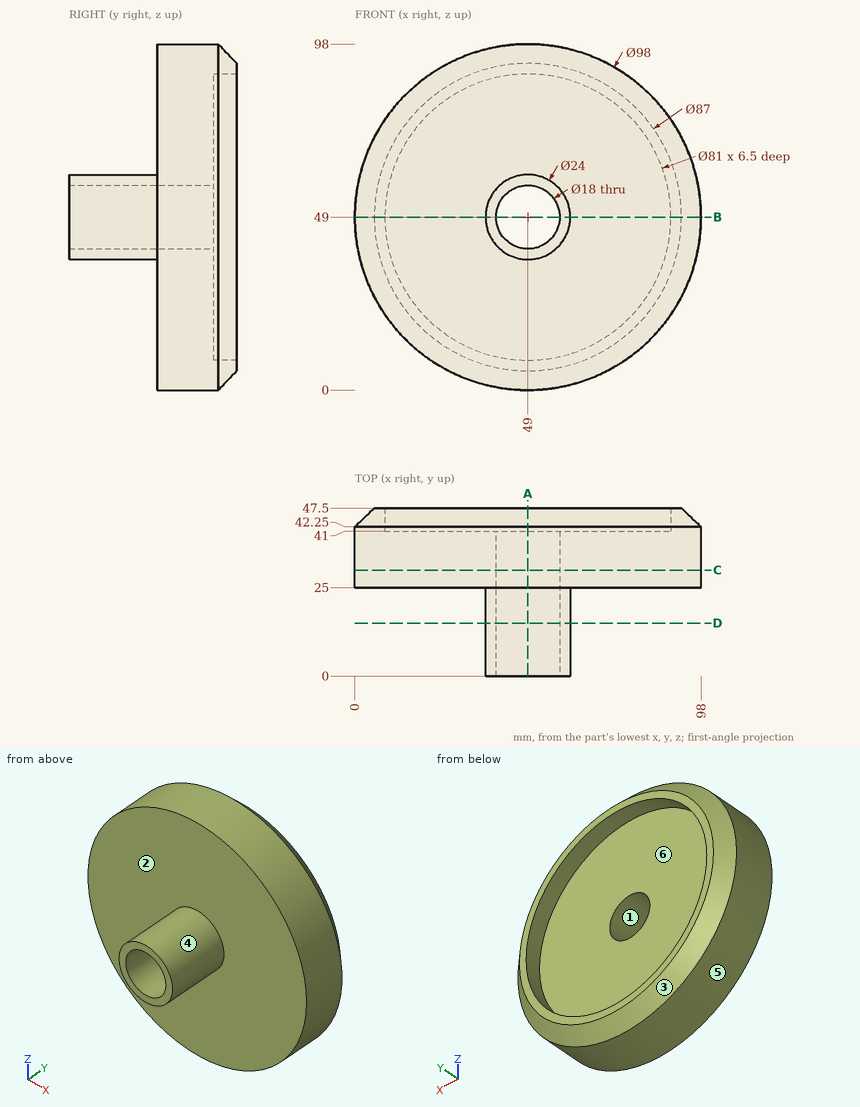
Source: three-view drawing plus pictorial views. Frame: mm from the lowest corner of the part. A direction names the side the tool comes from. Give positions to 0.01 mm unless a question says otherwise; leave off trailing zeros. Order: outer loops, then holes, each group sorted by start corner. A loop starts at its lowest first (then second) coordinate and runs counter-clockwise, first axis right, second up. Notation, with made-up numbers: (6.25, 36.25) -> (20.25, 36.25) arc R8 cw to (20.25, 44.25) -> close; hole circle Ø1 at (41, 70.25). An arc over 180 degrees is marked (long way). Write each question's results on one line, items separated by ' | '. Start each with the question number.
Item 1: Line query: line 1 (X direction, y = 42, z = 49); line 2 (X direction, y = 27, z = 49); line 3 (Y direction, x = 50, z = 64). Output: solid intervals per line, ascending.
Item 2: Cut plane C-C on y = 30. Return the cut outline in (x, z), then the cut area to 3 significant figures.
Item 3: Cut plane A-A on x = 49. Return the cut outline in (y, z).
Item 4: Contact query for flat-ended pins moving along their axis: P1, Ø1.5, axis at y = 27.5, z = 29, coming from the -X side; P2, Ø16, axis at x = 49, z = 49, coming from the +Y side; P3, Ø3, axis at x = 25.5, z = 37.5, coming from the -Y side; P4, Ø24.5, axis at x = 53.5, z = 40, coming from the +Y side. Output: stop coordinate, or through.
Item 5: Cut plane B-B on z = 49. Return the cut outline in (x, y), then the cut area to 3 significant figures.
Item 6: Set-up query: the marked faces 4, 5 and 6. Return all of +Z, -Z, +X, -X, +Y, -Y with unobstructed straight access to the full face (end or side cutting, diameter ignored); none if empty.
Item 7: Cut plane D-D on y = 15. Return the cut outline in (x, z).
Item 8: Mould query, pull axis Z, two halves, no side actions, for the marked faces 1, 2 and 3. Classes: pulls with the +Z half, pulls with the -Z half, needs draft (parallel to the pull), parting line crosses it, or undercut.
Established:
1) line 1: 0 to 8.5, 89.5 to 98 | line 2: 0 to 40, 58 to 98 | line 3: 25 to 41
2) outline: circle Ø98 at (49, 49); hole circle Ø18 at (49, 49) | area: 7,290 mm^2
3) outline: (0, 37) -> (25, 37) -> (25, 0) -> (42.25, 0) -> (47.5, 5.5) -> (47.5, 8.5) -> (41, 8.5) -> (41, 40) -> (0, 40) -> close; (0, 58) -> (41, 58) -> (41, 89.5) -> (47.5, 89.5) -> (47.5, 92.5) -> (42.25, 98) -> (25, 98) -> (25, 61) -> (0, 61) -> close
4) P1: x = 3.94 | P2: through | P3: y = 25 | P4: y = 41
5) outline: (0, 25) -> (37, 25) -> (37, 0) -> (40, 0) -> (40, 41) -> (8.5, 41) -> (8.5, 47.5) -> (5.5, 47.5) -> (0, 42.25) -> close; (58, 0) -> (61, 0) -> (61, 25) -> (98, 25) -> (98, 42.25) -> (92.5, 47.5) -> (89.5, 47.5) -> (89.5, 41) -> (58, 41) -> close | area: 1,510 mm^2
6) face 4: -Y | face 5: +Y, -Y | face 6: +Y
7) outline: circle Ø24 at (49, 49); hole circle Ø18 at (49, 49)
8) face 1: undercut | face 2: needs draft | face 3: parting line crosses it
